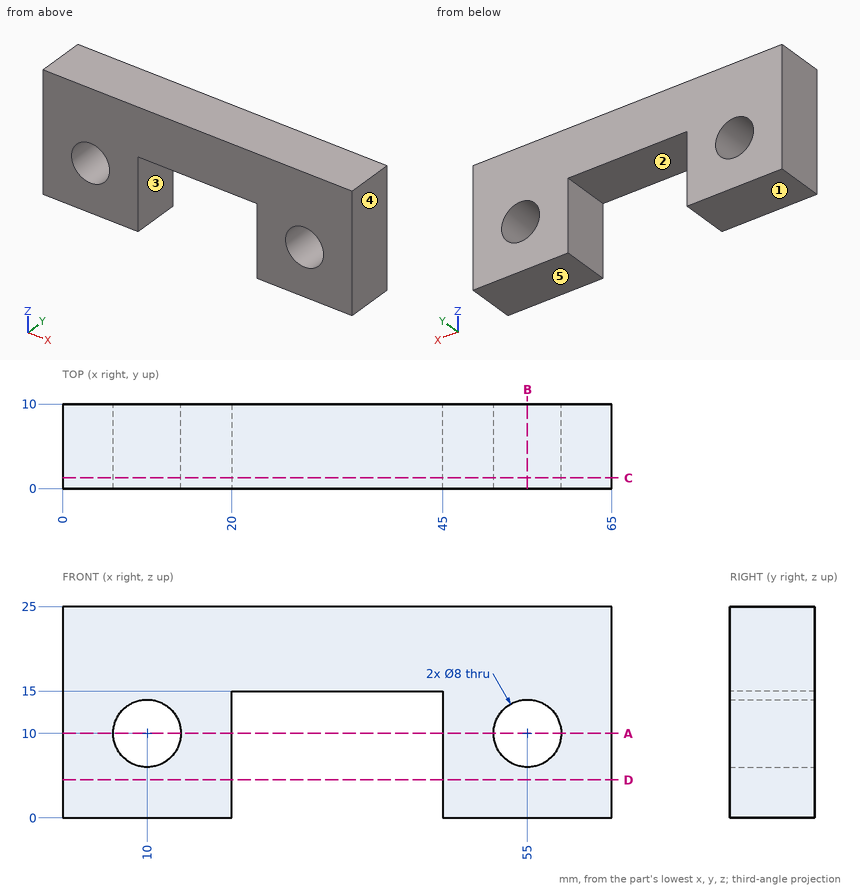
Here's the drawing with two shaded views (mm, measured from the low corner). I have some questions. A direction names the side the tool comes from. Coordinates: 2 decimals unless noted, no trailing zeros. Write each loop counter-clockwise with the first axis right and the second up, starting at its lowest first coordinate (ties: lowest second). Pieces come first, ordered by that corner, then holes. Notation, with made-up numbers: (83, -36) -> (107, -36) arc R18 ccw to (107, -8) -> close; hole circle Ø8 at (-22, 79). An arc over 180 degrees is marked (long way). One line per question, with ' | ' between items. Start each with the question number.
1. For the marked faces 1 and 2, which set-ups out of +Z, -Z, +X, -X, +Y, -Y let a thin tool reach every point of the face, with its end or its side?
2. If we section it at D-D (z = 4.5): Please give me the cut outline in (x, y).
3. Will this pin go through, and if not, where does the flat tip stop? P1, Ø2, axis at x = 39.5, y = 6.5, coming from the -Z side.
4. Thinking about a two-plate mould opening in X: for the marked faces 3, 4 and 5, which applies, pulls with the +X half, pulls with the -X half, needs draft (parallel to the pull), parting line crosses it, or undercut?
5. Please list where these lines run through material, in increasing order: line 1 along X through (y, z) = (6, 10); line 2 along X through (y, z) = (6.75, 9); line 3 along X through (y, z) = (3.25, 2.75).
6. If we section it at B-B (x = 55): Please give me the cut outline in (y, z).
7. If we section it at C-C (y = 1.25): Please give me the cut outline in (x, z), and give its area (3 significant figures).
8. If we section it at A-A (z = 10): Please give me the cut outline in (x, y), and give its area (3 significant figures).
Return value:
1) face 1: -Z, +X, -X, +Y, -Y | face 2: -Z, +Y, -Y
2) outline: (0, 0) -> (20, 0) -> (20, 10) -> (0, 10) -> close; (45, 0) -> (65, 0) -> (65, 10) -> (45, 10) -> close
3) P1: stops at z = 15
4) face 3: undercut | face 4: pulls with the +X half | face 5: needs draft
5) line 1: x = 0 to 6, 14 to 20, 45 to 51, 59 to 65 | line 2: x = 0 to 6.13, 13.87 to 20, 45 to 51.13, 58.87 to 65 | line 3: x = 0 to 20, 45 to 65
6) outline: (0, 0) -> (10, 0) -> (10, 6) -> (0, 6) -> close; (0, 14) -> (10, 14) -> (10, 25) -> (0, 25) -> close
7) outline: (0, 0) -> (20, 0) -> (20, 15) -> (45, 15) -> (45, 0) -> (65, 0) -> (65, 25) -> (0, 25) -> close; hole circle Ø8 at (10, 10); hole circle Ø8 at (55, 10) | area: 1,150 mm²
8) outline: (0, 0) -> (6, 0) -> (6, 10) -> (0, 10) -> close; (14, 0) -> (20, 0) -> (20, 10) -> (14, 10) -> close; (45, 0) -> (51, 0) -> (51, 10) -> (45, 10) -> close; (59, 0) -> (65, 0) -> (65, 10) -> (59, 10) -> close | area: 240 mm²
